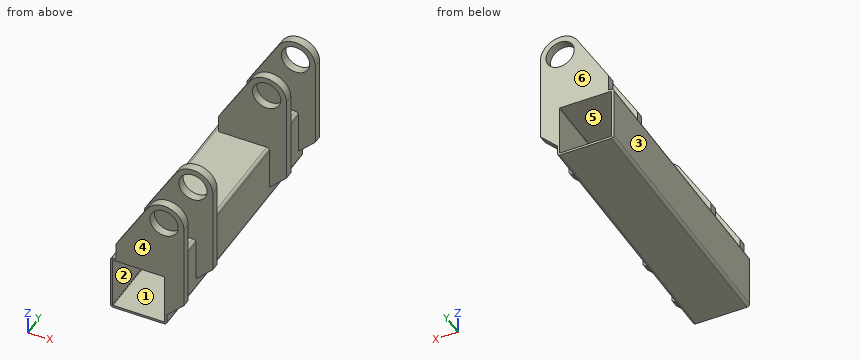
from build123d import *

# Parameters (mm, degrees)
F1_DEPTH = 235
F2_T     = -4
F0_R     = 25
F3_DEPTH = 15


with BuildPart() as f1:
    # F0 (on Front) → F1 (new body)
    with BuildSketch(Plane.XZ):
        with BuildLine():
            ThreePointArc((50, 45), (48.5355339059, 48.5355339059), (45, 50))
            Line((45, 50), (-40.3777472675, 50))
            Line((-40.3777472675, 50), (-45, 50))
            ThreePointArc((-45, 50), (-48.5355339059, 48.5355339059), (-50, 45))
            Line((-50, 45), (-50, -45))
            ThreePointArc((-50, -45), (-48.5355339059, -48.5355339059), (-45, -50))
            Line((-45, -50), (45, -50))
            ThreePointArc((45, -50), (48.5355339059, -48.5355339059), (50, -45))
            Line((50, -45), (50, -30))
            Line((50, -30), (50, 45))
        make_face()
    extrude(amount=-F1_DEPTH)

    # F2
    f2_openings = [f1.faces().sort_by_distance(p)[0] for p in [
        (0, 0, 0),
        (0, 235, 0),
    ]]
    offset(amount=F2_T, openings=f2_openings)

    # F0 (on Front) → F3 (join)
    with BuildSketch(Plane.XZ):
        with BuildLine():
            Line((-40.3777472675, 50), (45, 50))
            ThreePointArc((45, 50), (48.5355339059, 48.5355339059), (50, 45))
            Line((50, 45), (50, -30))
            Line((50, -30), (80, 0))
            Line((80, 0), (80, 155))
            ThreePointArc((80, 155), (54.2839853809, 188.7462237213), (14.9252791173, 172.9028255822))
            Line((14.9252791173, 172.9028255822), (-40.3777472675, 80))
            Line((-40.3777472675, 80), (-40.3777472675, 50))
        make_face()
        with Locations((45, 155)):
            Circle(F0_R, mode=Mode.SUBTRACT)
    extrude(amount=-F3_DEPTH)


with BuildPart() as f4_1:
    # F4: copy of F1
    add(f1.part.moved(Location((0, 100, 0))))


with BuildPart() as f1_1:
    add(f1.part)

    add(f4_1.part)  # F5 merges F4_1
    # F5: F1, F4_1 across face
    add(f1.part.mirror(Plane(origin=(0, 235, 0), x_dir=(1, 0, 0), z_dir=(0, 1, 0))))
    add(f4_1.part.mirror(Plane(origin=(0, 235, 0), x_dir=(1, 0, 0), z_dir=(0, 1, 0))))


solid = f1_1.part
For this review, take the finished solid that the model builds, in its own axes (mm). Face numbers are marked on the shaded views. A direction names the side the tool comes from. Round coordinates to 2 decimals unless told otherwise and drop trailing zeros. Loops run counter-clockwise (first coordinate to the right, second up) from the corner with the lowest first, then second, coordinate; pieces in that order, holes last. Notation, with made-up numbers: (-26.75, 4.25) - (30.25, 4.25) arc R20 cw to (30.25, 40.25) - close; hole circle Ø6 at (35, -10.5). An arc over 180 degrees is marked (long way). One line per item, written item: value. Start each with the question number.
Item 1: Clearance check with flat-ended pins moving along their axes: pin 1 Ø16.5 at (y, z) = (362, 66) entering from -X; pin 2 Ø6 at (x, y) = (49.5, 369.5) entering from +Z; pin 3 Ø4 at (y, z) = (97, 55) entering from +X (3 decimals). State where each tip first meets the part, or that it passes through.
Item 2: Take a section at A-A (z = 38.5). Give the boundary of the cut face in (x, y), plus the area to 3 significant figures.
Item 3: For L1, parallel to Y at x = -8, z = 134; L2, parallel to Z at x = 45, y = 463; L3, parallel to Z at x = 35, y = 159.5, list the stretches that pass through material, from the lowest coordinate up.
Item 4: Take a section at C-C (x = 63). State how many separate pieces and enclosed holes the cut face has, plus the area to 3 significant figures.
Item 5: Take a section at B-B (y = 189). Give the boundary of the cut face in (x, z), plus the area to 3 significant figures.
Item 6: For the marked faces 5 and 6, list the 3-axis set-ups (+Z, -Z, +X, -X, +Y, -Y) from which the entire face can be reached by the end or side of a thin tool; tool diameter is ignored.
Item 7: The part is to be moulded in two halves that separate along X. For the marked faces 1, 2, 3 and 4, say which applies: +X half, -X half, draft (parallel to the pull), parting line (faces both ways), or undercut.
Answer below:
1. pin 1: stops at x = -40.38
1. pin 2: stops at z = 189.97
1. pin 3: passes through
2. outline: (-50, 0) - (-46, 0) - (-46, 470) - (-50, 470) - close; (46, 0) - (80, 0) - (80, 15) - (50, 15) - (50, 100) - (80, 100) - (80, 115) - (50, 115) - (50, 355) - (80, 355) - (80, 370) - (50, 370) - (50, 455) - (80, 455) - (80, 470) - (46, 470) - close
2. area: 5,560 mm2
3. L1: y = 0 to 15, 100 to 115, 355 to 370, 455 to 470
3. L2: z = -50 to -46, 46 to 130, 180 to 190
3. L3: z = -50 to -46, 46 to 50
4. separate pieces: 8
4. enclosed holes: 0
4. area: 10,000 mm2
5. outline: (-50, -45) arc R5 ccw to (-45, -50) - (45, -50) arc R5 ccw to (50, -45) - (50, 45) arc R5 ccw to (45, 50) - (-45, 50) arc R5 ccw to (-50, 45) - close; hole (-46, -45) arc R1 ccw to (-45, -46) - (45, -46) arc R1 ccw to (46, -45) - (46, 45) arc R1 ccw to (45, 46) - (-45, 46) arc R1 ccw to (-46, 45) - close
5. area: 1,520 mm2
6. face 5: +Y, -Y
6. face 6: +Z, -Z, +X, -X, +Y
7. face 1: undercut
7. face 2: undercut
7. face 3: -X half
7. face 4: draft
